```python
from build123d import *

# Parameters (mm, degrees)
BOX053_W                  = 10
BOX053_H                  = 5
BOX053_DEPTH              = 10
BOX051_W                  = 29.6
BOX051_H                  = 2
BOX051_DEPTH              = 99.5
BOX046_W                  = 10
BOX046_H                  = 5
BOX046_DEPTH              = 10
CYLINDER005_R             = 3
CYLINDER005_DEPTH         = 10
BOX060_W                  = 56
BOX060_H                  = 10
BOX060_DEPTH              = 122
BOX050_W                  = 4
BOX050_H                  = 4.5
BOX050_DEPTH              = 8
BOX052_W                  = 17
BOX052_H                  = 7.5
BOX052_DEPTH              = 12.5
BOX044_W                  = 48.5
BOX044_H                  = 4.6
BOX044_DEPTH              = 25.5
FUSION016_PLACEMENT_ANGLE = 90
BOX048_W                  = 83.5
BOX048_H                  = 35.6
BOX048_DEPTH              = 8
BOX042_W                  = 114
BOX042_H                  = 50
BOX042_DEPTH              = 144
BOX041_W                  = 120
BOX041_H                  = 42
BOX041_DEPTH              = 150
BOX056_W                  = 72
BOX056_H                  = 18
BOX056_DEPTH              = 1.7
BOX047_W                  = 3
BOX047_H                  = 10
BOX047_DEPTH              = 5.8
ARRAY008_X_COUNT          = 2
ARRAY008_X_PITCH          = 67
BOX049_W                  = 77
BOX049_H                  = 10
BOX049_DEPTH              = 10
BOX055_W                  = 85.5
BOX055_H                  = 37.8
BOX055_DEPTH              = 8
CYLINDER004_R             = 1.2
CYLINDER004_DEPTH         = 4
CYLINDER003_R             = 2.6
CYLINDER003_DEPTH         = 4
ARRAY007_X_COUNT          = 2
ARRAY007_X_PITCH          = 25
ARRAY007_Z_COUNT          = 2
ARRAY007_Z_PITCH          = 95
BOX057_W                  = 10
BOX057_H                  = 77
BOX057_DEPTH              = 10
BOX045_W                  = 10
BOX045_H                  = 74
BOX045_DEPTH              = 10
CUT029_PLACEMENT_ANGLE    = 90
BOX058_W                  = 10
BOX058_H                  = 77
BOX058_DEPTH              = 10
BOX061_W                  = 10
BOX061_H                  = 74
BOX061_DEPTH              = 10
CUT028_PLACEMENT_ANGLE    = 90
BOX062_W                  = 10
BOX062_H                  = 77
BOX062_DEPTH              = 10
BOX059_W                  = 10
BOX059_H                  = 74
BOX059_DEPTH              = 10
CUT027_PLACEMENT_ANGLE    = 180
BOX054_W                  = 10
BOX054_H                  = 77
BOX054_DEPTH              = 10
BOX043_W                  = 10
BOX043_H                  = 74
BOX043_DEPTH              = 10
FILLET003_1_R             = 6
FILLET003_2_R             = 2
FILLET003_3_R             = 1


with BuildPart() as on_off001:
    # Box053 → Box053 (new body)
    with BuildSketch(Plane(origin=(26, -6, 81.5), x_dir=(1, 0, 0), z_dir=(0, 0, 1))):
        with Locations((5, 2.5)):
            Rectangle(BOX053_W, BOX053_H)
    extrude(amount=BOX053_DEPTH)


with BuildPart() as obj1:
    # Box051 → Box051 (new body)
    with BuildSketch(Plane.XY):
        with Locations((14.8, 1)):
            Rectangle(BOX051_W, BOX051_H)
    extrude(amount=BOX051_DEPTH)


with BuildPart() as obj2:
    # Box046 → Box046 (new body)
    with BuildSketch(Plane(origin=(26, 0.6, 5.5), x_dir=(1, 0, 0), z_dir=(0, 0, 1))):
        with Locations((5, 2.5)):
            Rectangle(BOX046_W, BOX046_H)
    extrude(amount=BOX046_DEPTH)

    # Fusion017: union on_off001, obj1
    add(on_off001.part)
    add(obj1.part)


with BuildPart() as obj2_1:
    # Fusion017 placement: moved
    add(obj2.part.moved(Location((85.8, 76, 19.23))))


with BuildPart() as obj3:
    # Cylinder005 → Cylinder005 (new body)
    with BuildSketch(Plane(origin=(101.22, 63.68, 142.21), x_dir=(1, 0, 0), z_dir=(0, 0, 1))):
        Circle(CYLINDER005_R)
    extrude(amount=CYLINDER005_DEPTH)


with BuildPart() as obj4:
    # Box060 → Box060 (new body)
    with BuildSketch(Plane(origin=(11, 81, 19), x_dir=(1, 0, 0), z_dir=(0, 0, 1))):
        with Locations((28, 5)):
            Rectangle(BOX060_W, BOX060_H)
    extrude(amount=BOX060_DEPTH)


with BuildPart() as obj5:
    # Box050 → Box050 (new body)
    with BuildSketch(Plane(origin=(83, 15.25, 0), x_dir=(1, 0, 0), z_dir=(0, 0, 1))):
        with Locations((2, 2.25)):
            Rectangle(BOX050_W, BOX050_H)
    extrude(amount=BOX050_DEPTH)


with BuildPart() as cubo029:
    # Box052 → Box052 (new body)
    with BuildSketch(Plane(origin=(-7, 2.4, 6.55), x_dir=(1, 0, 0), z_dir=(0, 0, 1))):
        with Locations((8.5, 3.75)):
            Rectangle(BOX052_W, BOX052_H)
    extrude(amount=BOX052_DEPTH)


with BuildPart() as obj6:
    # Box044 → Box044 (new body)
    with BuildSketch(Plane(origin=(0, 0.4, 0), x_dir=(1, 0, 0), z_dir=(0, 0, 1))):
        with Locations((24.25, 2.3)):
            Rectangle(BOX044_W, BOX044_H)
    extrude(amount=BOX044_DEPTH)

    # Fusion016: union Cubo029
    add(cubo029.part)


with BuildPart() as obj6_1:
    # Fusion016 placement: moved
    add(obj6.part.moved(Location((0, 30.25, 7.6))).rotate(Axis((0, 30.25, 7.6), (1, 0, 0)), FUSION016_PLACEMENT_ANGLE))


with BuildPart() as fusion013:
    # Box048 → Box048 (new body)
    with BuildSketch(Plane.XY):
        with Locations((41.75, 17.8)):
            Rectangle(BOX048_W, BOX048_H)
    extrude(amount=BOX048_DEPTH)

    # Fusion014: union obj5, obj6
    add(obj5.part)
    add(obj6_1.part)


with BuildPart() as fusion013_1:
    # Fusion014 placement: moved
    add(fusion013.part.moved(Location((3, 46.4, 3))))

    # Fusion013: union obj2, obj3, obj4
    add(obj2_1.part)
    add(obj3.part)
    add(obj4.part)


with BuildPart() as cubo023:
    # Box042 → Box042 (new body)
    with BuildSketch(Plane(origin=(3, 32, 3), x_dir=(1, 0, 0), z_dir=(0, 0, 1))):
        with Locations((57, 25)):
            Rectangle(BOX042_W, BOX042_H)
    extrude(amount=BOX042_DEPTH)


with BuildPart() as cut024:
    # Box041 → Box041 (new body)
    with BuildSketch(Plane(origin=(0, 42, 0), x_dir=(1, 0, 0), z_dir=(0, 0, 1))):
        with Locations((60, 21)):
            Rectangle(BOX041_W, BOX041_H)
    extrude(amount=BOX041_DEPTH)

    # Cut024: cut Cubo023
    add(cubo023.part, mode=Mode.SUBTRACT)


with BuildPart() as leds002:
    # Box056 → Box056 (new body)
    with BuildSketch(Plane(origin=(-1, 0, 2), x_dir=(1, 0, 0), z_dir=(0, 0, 1))):
        with Locations((36, 9)):
            Rectangle(BOX056_W, BOX056_H)
    extrude(amount=BOX056_DEPTH)


with BuildPart() as soporte_placa_leds001:
    # Box047 → Box047 (new body)
    with BuildSketch(Plane(origin=(0, 8, 0), x_dir=(1, 0, 0), z_dir=(0, 0, 1))):
        with Locations((1.5, 5)):
            Rectangle(BOX047_W, BOX047_H)
    extrude(amount=BOX047_DEPTH)

    # Array008 X: soporte_placa_leds001 ×2


with BuildPart() as soporte_placa_leds001_1:
    add(soporte_placa_leds001.part)
    with Locations(*[(i * ARRAY008_X_PITCH, 0, 0) for i in range(1, ARRAY008_X_COUNT)]):
        add(soporte_placa_leds001.part)

    # Cut023: cut leds002
    add(leds002.part, mode=Mode.SUBTRACT)


with BuildPart() as soporte_placa_leds001_2:
    # Cut023 placement: moved
    add(soporte_placa_leds001_1.part.moved(Location((4, 65, 70.25))))


with BuildPart() as cubo028:
    # Box049 → Box049 (new body)
    with BuildSketch(Plane(origin=(9, 43, 3), x_dir=(1, 0, 0), z_dir=(0, 0, 1))):
        with Locations((38.5, 5)):
            Rectangle(BOX049_W, BOX049_H)
    extrude(amount=BOX049_DEPTH)


with BuildPart() as baseproto001:
    # Box055 → Box055 (new body)
    with BuildSketch(Plane(origin=(3, 44.2, 3), x_dir=(1, 0, 0), z_dir=(0, 0, 1))):
        with Locations((42.75, 18.9)):
            Rectangle(BOX055_W, BOX055_H)
    extrude(amount=BOX055_DEPTH)

    # Cut030: cut Cubo028
    add(cubo028.part, mode=Mode.SUBTRACT)


with BuildPart() as cilindro004:
    # Cylinder004 → Cylinder004 (new body)
    with BuildSketch(Plane(origin=(2.6, 0, 2.6), x_dir=(1, 0, 0), z_dir=(0, -1, 0))):
        Circle(CYLINDER004_R)
    extrude(amount=CYLINDER004_DEPTH)


with BuildPart() as obj7:
    # Cylinder003 → Cylinder003 (new body)
    with BuildSketch(Plane(origin=(2.6, 0, 2.6), x_dir=(1, 0, 0), z_dir=(0, -1, 0))):
        Circle(CYLINDER003_R)
    extrude(amount=CYLINDER003_DEPTH)

    # Cut025: cut Cilindro004
    add(cilindro004.part, mode=Mode.SUBTRACT)


with BuildPart() as obj7_1:
    # Cut025 placement: moved
    add(obj7.part.moved(Location((31.199794, 82, -20.171414))))

    # Array007 X: obj7_2


with BuildPart() as obj7_2:
    add(obj7_1.part)
    with Locations(*[(i * ARRAY007_X_PITCH, 0, 0) for i in range(1, ARRAY007_X_COUNT)]):
        add(obj7_1.part)

    # Array007 Z: obj7_2


with BuildPart() as obj7_3:
    add(obj7_2.part)
    with Locations(*[(0, 0, i * ARRAY007_Z_PITCH) for i in range(1, ARRAY007_Z_COUNT)]):
        add(obj7_2.part)


with BuildPart() as obj7_4:
    # Array007 placement: moved
    add(obj7_3.part.moved(Location((54.6, 0, 39))))


with BuildPart() as cubo031:
    # Box057 → Box057 (new body)
    with BuildSketch(Plane(origin=(0, 10, 140), x_dir=(1, 0, 0), z_dir=(0, 0, 1))):
        with Locations((5, 38.5)):
            Rectangle(BOX057_W, BOX057_H)
    extrude(amount=BOX057_DEPTH)


with BuildPart() as cut029:
    # Box045 → Box045 (new body)
    with BuildSketch(Plane(origin=(-3, 10, 143), x_dir=(1, 0, 0), z_dir=(0, 0, 1))):
        with Locations((5, 37)):
            Rectangle(BOX045_W, BOX045_H)
    extrude(amount=BOX045_DEPTH)

    # Cut029: cut Cubo031
    add(cubo031.part, mode=Mode.SUBTRACT)


with BuildPart() as cut029_1:
    # Cut029 placement: moved
    add(cut029.part.moved(Location((-30, 0, 150))).rotate(Axis((-30, 0, 150), (0, 1, 0)), CUT029_PLACEMENT_ANGLE))


with BuildPart() as cubo032:
    # Box058 → Box058 (new body)
    with BuildSketch(Plane(origin=(0, 10, 140), x_dir=(1, 0, 0), z_dir=(0, 0, 1))):
        with Locations((5, 38.5)):
            Rectangle(BOX058_W, BOX058_H)
    extrude(amount=BOX058_DEPTH)


with BuildPart() as cut028:
    # Box061 → Box061 (new body)
    with BuildSketch(Plane(origin=(-3, 10, 143), x_dir=(1, 0, 0), z_dir=(0, 0, 1))):
        with Locations((5, 37)):
            Rectangle(BOX061_W, BOX061_H)
    extrude(amount=BOX061_DEPTH)

    # Cut028: cut Cubo032
    add(cubo032.part, mode=Mode.SUBTRACT)


with BuildPart() as cut028_1:
    # Cut028 placement: moved
    add(cut028.part.moved(Location((150, 0, 0))).rotate(Axis((150, 0, 0), (0, -1, 0)), CUT028_PLACEMENT_ANGLE))


with BuildPart() as cubo035:
    # Box062 → Box062 (new body)
    with BuildSketch(Plane(origin=(0, 10, 140), x_dir=(1, 0, 0), z_dir=(0, 0, 1))):
        with Locations((5, 38.5)):
            Rectangle(BOX062_W, BOX062_H)
    extrude(amount=BOX062_DEPTH)


with BuildPart() as cut027:
    # Box059 → Box059 (new body)
    with BuildSketch(Plane(origin=(-3, 10, 143), x_dir=(1, 0, 0), z_dir=(0, 0, 1))):
        with Locations((5, 37)):
            Rectangle(BOX059_W, BOX059_H)
    extrude(amount=BOX059_DEPTH)

    # Cut027: cut Cubo035
    add(cubo035.part, mode=Mode.SUBTRACT)


with BuildPart() as cut027_1:
    # Cut027 placement: moved
    add(cut027.part.moved(Location((120, 0, 150))).rotate(Axis((120, 0, 150), (0, 1, 0)), CUT027_PLACEMENT_ANGLE))


with BuildPart() as cubo030:
    # Box054 → Box054 (new body)
    with BuildSketch(Plane(origin=(0, 10, 140), x_dir=(1, 0, 0), z_dir=(0, 0, 1))):
        with Locations((5, 38.5)):
            Rectangle(BOX054_W, BOX054_H)
    extrude(amount=BOX054_DEPTH)


with BuildPart() as closet_bottom_generic:
    # Box043 → Box043 (new body)
    with BuildSketch(Plane(origin=(-3, 10, 143), x_dir=(1, 0, 0), z_dir=(0, 0, 1))):
        with Locations((5, 37)):
            Rectangle(BOX043_W, BOX043_H)
    extrude(amount=BOX043_DEPTH)

    # Cut026: cut Cubo030
    add(cubo030.part, mode=Mode.SUBTRACT)

    # Fusion015: union Cut029, Cut028, Cut027
    add(cut029_1.part)
    add(cut028_1.part)
    add(cut027_1.part)

    # Fusion012: union Cut024, soporte_placa_leds001, baseProto001, obj7
    add(cut024.part)
    add(soporte_placa_leds001_2.part)
    add(baseproto001.part)
    add(obj7_4.part)

    # Cut022: cut Fusion013
    add(fusion013_1.part, mode=Mode.SUBTRACT)

    # Fillet003 1
    fillet003_1_edges = [closet_bottom_generic.edges().sort_by_distance(p)[0] for p in [
        (88.5, 52.925, 3),
        (88.5, 74.075, 3),
        (5.5, 82, 70.25),
        (5.5, 82, 76.05),
        (72.5, 82, 70.25),
        (72.5, 82, 76.05),
    ]]
    fillet(fillet003_1_edges, radius=FILLET003_1_R)

    # Fillet003 2
    fillet003_2_edges = [closet_bottom_generic.edges().sort_by_distance(p)[0] for p in [
        (6, 44.2, 3),
    ]]
    fillet(fillet003_2_edges, radius=FILLET003_2_R)

    # Fillet003 3
    fillet003_3_edges = [closet_bottom_generic.edges().sort_by_distance(p)[0] for p in [
        (0, 57.6, 16.75),
        (0, 63.85, 13),
        (0, 70.1, 16.75),
        (0, 63.85, 20.5),
        (120, 79.1, 34.73),
        (120, 76.6, 29.73),
        (120, 79.1, 24.73),
        (120, 81.6, 29.73),
        (120, 72.5, 100.73),
        (120, 75, 105.73),
        (120, 72.5, 110.73),
        (120, 70, 105.73),
        (85.799794, 82, 21.428586),
        (110.799794, 82, 21.428586),
        (85.799794, 82, 116.428586),
        (110.799794, 82, 116.428586),
    ]]
    fillet(fillet003_3_edges, radius=FILLET003_3_R)


solid = closet_bottom_generic.part
```
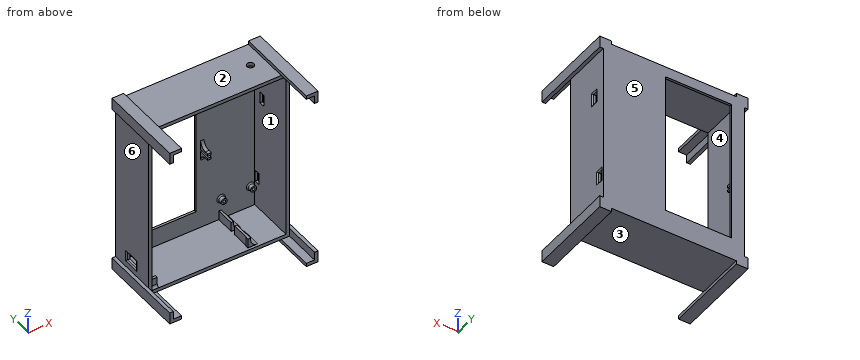
Verification items for the finished model (mm, model axes). Face numbers are marked on the shaded views. A direction names the side the tool comes from. Give positions to 0.01 mm unless a question says otherwise; leave off trailing zeros. Order: outer loops, then holes, each group sorted by start corner. A loop starts at its lowest first (then second) coordinate and runs counter-clockwise, first axis right, second up. Notation, with made-up numbers: M 67,42.5 L 83,42.5 A14 ccw 83,66.5 Z; hole C -6,58 d9. An arc over 180 degrees is marked long. Return JSON: item names as keys, results as strings. Group by question number.
1) Section check C-C on z = 139. Record the cut outline in (x, y), and give its area (3 significant figures).
2) Go/stop test with flat-tipped pins: pin 1 Ø12 at (x, y) = (81, 68) entering from -Z; pin 2 Ø12 at (x, y) = (26.5, 46.5) entering from +Z; pin 3 Ø5 at (y, z) = (64, 45.5) entering from +X; pin 4 Ø10 at (x, z) = (19.5, 113.5) entering from -Y. Record where each tip stops, or that it passes through.
3) Scan lines: line 1 (X direction, y = 51.5, z = 37); line 2 (Z direction, x = 11, y = 74); line 3 (Z direction, x = 115.5, y = 27). Record each from-to range of solid material in increasing order.
4) Section check A-A on x = 27.5. Record the cut outline in (y, z), and give its area (3 significant figures).
5) Mould release check, pull along X, two halves, no side actions. Record for the marked faces 4, 5 and 6: pulls with the +X half, pulls with the -X half, needs draft (parallel to the pull), parting line crosses it, or undercut.
6) Access from +Z, -Z, +X, -X, +Y, -Y to the whole of each face (thin tool, end or side, straight path). Record for the marked faces 1, 2 and 3.
Answer block:
{
 "1": {"outline": "M 0,42 L 3,42 L 3,82 L 11,82 L 11,84 L 0,84 Z; M 67,82 L 117,82 L 117,42 L 120,42 L 120,84 L 67,84 Z", "area": "368 mm^2"},
 "2": {"pin 1": "stops at z = 0", "pin 2": "stops at z = 150", "pin 3": "stops at x = 120", "pin 4": "passes through"},
 "3": {"line 1": "x = 0 to 3, 117 to 120", "line 2": "z = 0 to 3, 147 to 150", "line 3": "z = -3 to 0, 150 to 153"},
 "4": {"outline": "M 42,0 L 84,0 L 84,19 L 82,19 L 82,3 L 42,3 Z; M 42,147 L 82,147 L 82,141 L 84,141 L 84,150 L 42,150 Z", "area": "296 mm^2"},
 "5": {"face 4": "undercut", "face 5": "needs draft", "face 6": "pulls with the -X half"},
 "6": {"face 1": "-Y", "face 2": "+Z, +Y, -Y", "face 3": "-Z, +Y, -Y"}
}
